```python
from build123d import *

# Parameters (mm, degrees)
SM_BASE_FLANGE_1_DEPTH      = 24
SM_EDGE_FLANGE_1_DEPTH      = 345.238328462
SM_EDGE_FLANGE_1_BEND_DEPTH = 345.238328462
HOLE_WIZARD_M4_3_D          = 4.3
HOLE_WIZARD_M4_4_D          = 4.3


# Sheet-metal steps are written as plain solids
with BuildPart() as part:
    # Sketch 1 → 基体-法兰1 (new, symmetric)
    with BuildSketch(Plane(origin=(0, 0, 0), x_dir=(1, 0, 0), z_dir=(0, 1, 0))):
        with BuildLine():
            Line((63, 329), (63, 320.299307498))
            ThreePointArc((63, 320.299307498), (63.028998532, 320.005786319), (63.11487291, 319.723614051))
            Line((63.11487291, 319.723614051), (195.615835089, 0.924306553))
            ThreePointArc((195.615835089, 0.924306553), (196.168357882, 0.252294071), (197.000962179, 0))
            Line((197.000962179, 0), (214, 0))
            Line((214, 0), (214, -1.5))
            Line((214, -1.5), (197.000962179, -1.5))
            ThreePointArc((197.000962179, -1.5), (195.335753585, -0.995411858), (194.230707999, 0.348613106))
            Line((194.230707999, 0.348613106), (61.72974582, 319.147920604))
            ThreePointArc((61.72974582, 319.147920604), (61.557997065, 319.71226514), (61.5, 320.299307498))
            Line((61.5, 320.299307498), (61.5, 329))
            Line((61.5, 329), (63, 329))
        make_face()
    extrude(amount=SM_BASE_FLANGE_1_DEPTH, both=True)

    # 边线-法兰1 section (across the edge) → 边线-法兰1 (add)
    with BuildSketch(Plane(origin=(194.230707999, 25.5, -0.348613106), x_dir=(0, -1, 0), z_dir=(-0.3837956311773727, 0, -0.9234180599756332))):
        with BuildLine():
            Line((-1.5, 1.5), (-1.5, 8))
            Line((-1.5, 8), (0, 8))
            Line((0, 8), (0, 1.5))
            ThreePointArc((0, 1.5), (0.439339828, 0.439339828), (1.5, 0))
            Line((1.5, 0), (1.5, -1.5))
            ThreePointArc((1.5, -1.5), (-0.621320344, -0.621320344), (-1.5, 1.5))
        make_face()
    extrude(amount=SM_EDGE_FLANGE_1_DEPTH)

    # 边线-法兰1 section 2 (across the edge) → 边线-法兰1 bend (add)
    with BuildSketch(Plane(origin=(61.72974582, -25.5, -319.147920604), x_dir=(0, 1, 0), z_dir=(0.3837956311773727, 0, 0.9234180599756332))):
        with BuildLine():
            Line((-1.5, 1.5), (-1.5, 8))
            Line((-1.5, 8), (0, 8))
            Line((0, 8), (0, 1.5))
            ThreePointArc((0, 1.5), (0.439339828, 0.439339828), (1.5, 0))
            Line((1.5, 0), (1.5, -1.5))
            ThreePointArc((1.5, -1.5), (-0.621320344, -0.621320344), (-1.5, 1.5))
        make_face()
    extrude(amount=SM_EDGE_FLANGE_1_BEND_DEPTH)

    # M4 间隙槽口3 (through all)
    with Locations(Plane(origin=(63, 0, 0), x_dir=(0, 0, -1), z_dir=(1, 0, 0))):
        with Locations((325, 14), (325, -14)):
            Hole(HOLE_WIZARD_M4_3_D / 2)

    # M4 间隙槽口4 (through all)
    with Locations(Plane(origin=(0, 0, 0), x_dir=(-1, 0, 0), z_dir=(0, 0, -1))):
        with Locations((-205, 14), (-205, -14)):
            Hole(HOLE_WIZARD_M4_4_D / 2)


solid = part.part
```
The listing builds one solid part. Answer for the finished solid, in the listing's coordinates (mm). A direction names the side the tool comes from. Coordinates: 2 decimals unless noted, no trailing zeros. Write each loop counter-clockwise with the first axis right and the second up, starting at its lowest first coordinate (ties: lowest second). Pieces come first, ordered by that corner, then holes. Notation, with made-up numbers: (-35.75, -3.5) - (11.25, -3.5) arc R17 cw to (11.25, 23.5) - close; hole circle Ø7 at (37, 11.25). An arc over 180 degrees is marked (long way). Return JSON: item names as keys, results as strings. Group by question number.
1. Determine the mould class of faces 4 (the flat face through (123, -27, -160)), 5 (the cylindrical face through (126.64, -25.07, -161.81)), 6 (the flat face through (206, 0, 1.5)), 7 (the flat face through (125, 27, -156)) for opening direction Y: released by +Y, released by -Y, zero draft, split by the parting line, or undercut.
2. Given pin 1 (7 mm diameter, centred on y = 14, z = -325, fed in from +X); pin 2 (5 mm diameter, centred on y = 15.5, z = -234, fed in from +X); pin 3 (3 mm diameter, centred on y = 13.5, z = -188, fed in from +X), each flat-ended and moving along its own axis, determine where each tip first touches the part or whether it passes through.
3. Which of the six approach directions +Z, -Z, +X, -X, +Y, -Y give full straight-line access (tool end or side, diameter ignored) to faces 1 (the flat face through (123, -25.5, -160)), 2 (the flat face through (205, 0, 0)), 3 (the flat face through (61.5, 0, -325))?
4. A cutting plane is placed at A-A, the plane y = 6.5. Determine the outline of the cut face in (x, z), plus the area to 3 significant figures.
5. Straight lines are drawn through the part: L1, parallel to Y at x = 62.1, z = -325; L2, parallel to Y at x = 146, z = -104; L3, parallel to X at y = 3.5, z = -243. For each, find the intervals that lie inside material, in ascending order.
Ans:
{
 "1": {"face 4": "released by -Y", "face 5": "undercut", "face 6": "zero draft", "face 7": "released by +Y"},
 "2": {"pin 1": "x = 63", "pin 2": "x = 99.78", "pin 3": "x = 118.49"},
 "3": {"face 1": "+Z, -X", "face 2": "-Z, +X, +Y, -Y", "face 3": "+Z, -Z, -X, +Y, -Y"},
 "4": {"outline": "(61.5, -329) - (63, -329) - (63, -320.3) arc R1.5 cw to (63.11, -319.72) - (195.62, -0.92) arc R1.5 cw to (197, 0) - (214, 0) - (214, 1.5) - (197, 1.5) arc R3 ccw to (194.23, -0.35) - (61.73, -319.15) arc R3 ccw to (61.5, -320.3) - close", "area": "562 mm²"},
 "5": {"L1": "-24 to -16.15, -11.85 to 11.85, 16.15 to 24", "L2": "-27 to -25.5, 25.5 to 27", "L3": "93.38 to 95"}
}
